from build123d import *

# Parameters (mm, degrees)
BASE_EXTRUDE_DEPTH = 6
HOLE1_START        = 9
HOLE1_OUTLINE_R    = 5
HOLE1_DEPTH        = 6


# Read off the part's stored shape, not the designer's step: Hole1
with BuildPart() as part:
    # Sketch1 → Base-Extrude (new body)
    with BuildSketch(Plane(origin=(0, 0, 15), x_dir=(-1, 0, 0), z_dir=(0, 0, -1))):
        with BuildLine():
            Line((-35.94095366, -10), (-34.656774357, 8.985563209))
            ThreePointArc((-34.656774357, 8.985563209), (-32.674273273, 15.485526346), (-28.02703118, 20.443648194))
            Line((-28.02703118, 20.443648194), (-16.313883273, 28.273529827))
            Line((-16.313883273, 28.273529827), (-38.001708808, 60.717533475))
            ThreePointArc((-38.001708808, 60.717533475), (-50.661713644, 64.166190146), (-55.838522693, 52.109258389))
            Line((-55.838522693, 52.109258389), (-35.94095366, -10))
        make_face()
    extrude(amount=BASE_EXTRUDE_DEPTH)

    # Hole1 outline → Hole1 (cut)
    with BuildSketch(Plane.XY.offset(HOLE1_START)):
        with Locations((46.315287905, 55.160159761)):
            Circle(HOLE1_OUTLINE_R)
    extrude(amount=HOLE1_DEPTH, mode=Mode.SUBTRACT)


solid = part.part
CAD build for the part. Positions are in the model's coordinates, mm. Give positions to 0.01 mm unless a question says otherwise; leave off trailing zeros. Write each loop counter-clockwise with the first axis right and the second up, starting at its lowest first coordinate (ties: lowest second). Pieces come first, ordered by that corner, then holes. Notation, with made-up numbers: (58.5, 87) - (70.5, 87) arc R19 ccw to (70.5, 120) - close; hole circle Ø4 at (28, 53). An arc over 180 degrees is marked (long way). Put each result on its own line as item: value.
(1) Wall check: L1, parallel to X at y = 17, z = 11.05; L2, parallel to X at y = -1.5, z = 14.7; L3, parallel to X at y = 59, z = 12.6. Give the ranges that are in metal, low to high.
Working result:
L1: 31.67 to 44.59
L2: 35.37 to 38.66
L3: 36.85 to 43.11, 49.52 to 55.55
(2) Saw through at A-A (z = 13). List the corners of the cut face in (x, y).
Working result:
outline: (16.31, 28.27) - (28.03, 20.44) arc R15 cw to (34.66, 8.99) - (35.94, -10) - (55.84, 52.11) arc R10 ccw to (38, 60.72) - close; hole circle Ø10 at (46.32, 55.16)
(3) Saw through at B-B (y = 25). List the corners of the cut face in (x, z), then the cut area to 3 significant figures.
Working result:
outline: (21.21, 9) - (47.15, 9) - (47.15, 15) - (21.21, 15) - close
area: 156 mm^2
(4) Saw through at C-C (x = 24). List the corners of the cut face in (y, z), then the cut area to 3 significant figures.
Working result:
outline: (23.14, 9) - (39.77, 9) - (39.77, 15) - (23.14, 15) - close
area: 99.8 mm^2
(5) Pull direction Y, two halves, no side cores. Call faces 1 (the cylindrical face through (32.722, 15.402, 12.042)), 2 (the cylindrical face through (42.63, 58.54, 11.96)), 3 (the flat face through (27.006, 44.268, 12.042)): released by +Y, released by -Y, zero draft, split by the parting line, or undercut.
Working result:
face 1: released by -Y
face 2: undercut
face 3: released by +Y
(6) Drop flat-ended pins along their axis: pin 1 Ø1 at (y, z) = (19, 12.5) entering from +X; pin 2 Ø3 at (y, z) = (42.5, 13) entering from -X; pin 3 Ø1 at (y, z) = (26, 10.5) entering from -X; pin 4 Ø6 at (x, y) = (46.32, 55.16) entering from +Z. Give the stop position or say it passes through.
Working result:
pin 1: x = 45.39
pin 2: x = 24.82
pin 3: x = 18.97
pin 4: through
